Read the model definition and answer for the solid it produces. Units are mm, in the model's axes. Face numbers are marked on the shaded views. A direction names the side the tool comes from. Coordinates: 2 decimals unless noted, no trailing zeros. Loops run counter-clockwise (first coordinate to the right, second up) from the corner with the lowest first, then second, coordinate; pieces in that order, holes last.
from build123d import *

# Parameters (mm, degrees)
SKETCH1_R           = 18.5
BOSS_EXTRUDE1_DEPTH = 68
SKETCH3_R           = 6
BOSS_EXTRUDE2_DEPTH = 3.5
SKETCH4_R           = 3
BOSS_EXTRUDE3_DEPTH = 10.4
CUT_EXTRUDE1_START  = -8
CUT_EXTRUDE1_DEPTH  = 8


with BuildPart() as part:
    # Sketch1 → Boss-Extrude1 (new body)
    with BuildSketch(Plane.XY):
        Circle(SKETCH1_R)
    extrude(amount=BOSS_EXTRUDE1_DEPTH)

    # Sketch3 → Boss-Extrude2 (add)
    with BuildSketch(Plane.XY):
        Circle(SKETCH3_R)
    extrude(amount=-BOSS_EXTRUDE2_DEPTH)

    # Sketch4 → Boss-Extrude3 (add)
    with BuildSketch(Plane(origin=(0, 0, -3.5), x_dir=(-1, 0, 0), z_dir=(0, 0, -1))):
        Circle(SKETCH4_R)
    extrude(amount=BOSS_EXTRUDE3_DEPTH)

    # Sketch5 → Cut-Extrude1 (cut)
    with BuildSketch(Plane(origin=(0, 0, -13.9), x_dir=(-1, 0, 0), z_dir=(0, 0, -1)).offset(CUT_EXTRUDE1_START)):
        with BuildLine():
            Line((-2.236067977, 2), (2.236067977, 2))
            ThreePointArc((2.236067977, 2), (0, 3), (-2.236067977, 2))
        make_face()
    extrude(amount=CUT_EXTRUDE1_DEPTH, mode=Mode.SUBTRACT)


solid = part.part
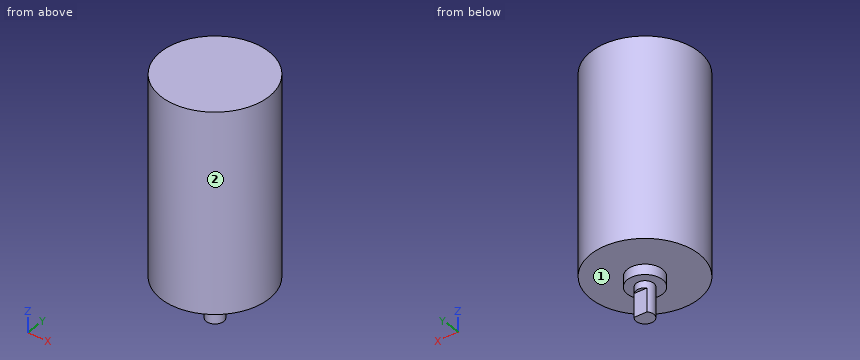
Item 1: Find the intervals of material crossed by line 1 along Z through (x, y) = (9, -4.5); line 2 along Y through (x, z) = (13, 50); line 3 along Y through (x, z) = (-9, 33), in increasing order.
Numbers:
line 1: z = 0 to 68
line 2: y = -13.16 to 13.16
line 3: y = -16.16 to 16.16
Item 2: A cutting plane is placed at A-A on x = 0. Determine the outline of the cut face in (y, z).
Numbers:
outline: (-18.5, 0) - (-6, 0) - (-6, -3.5) - (-3, -3.5) - (-3, -13.9) - (2, -13.9) - (2, -5.9) - (3, -5.9) - (3, -3.5) - (6, -3.5) - (6, 0) - (18.5, 0) - (18.5, 68) - (-18.5, 68) - close
Item 3: Which of the six approach directions +Z, -Z, +X, -X, +Y, -Y give full straight-line access (tool end or side, diameter ignored) to the marked faces 1 and 2?
Numbers:
face 1: -Z
face 2: +Z, -Z
Item 4: Given pin 1 (0.8 mm diameter, centred on x = -0.5, y = 2.5, fed in from -Z); pin 2 (8 mm diameter, centred on y = 12.5, z = -2, fed in from -X); pin 3 (8 mm diameter, centred on x = -7, y = 5.5, fed in from -Z), each flat-ended and moving along its own axis, determine where each tip first touches the part or whether it passes through.
Numbers:
pin 1: stops at z = -5.9
pin 2: stops at x = -16.14
pin 3: stops at z = -3.5
Item 5: A cutting plane is placed at C-C on z = 18. Determine the outline of the cut face in (x, y), then the cut area to 3 significant figures.
Numbers:
outline: circle Ø37 at (0, 0)
area: 1,080 mm2
Item 6: A cutting plane is placed at D-D on z = -4.5. Determine the outline of the cut face in (x, y), then the cut area to 3 significant figures.
Numbers:
outline: circle Ø6 at (0, 0)
area: 28.3 mm2
Item 7: A cutting plane is placed at B-B on y = 0. Determine the outline of the cut face in (x, z).
Numbers:
outline: (-18.5, 0) - (-6, 0) - (-6, -3.5) - (-3, -3.5) - (-3, -13.9) - (3, -13.9) - (3, -3.5) - (6, -3.5) - (6, 0) - (18.5, 0) - (18.5, 68) - (-18.5, 68) - close
